Geometry: final body of the model. Coordinates: model frame, mm. Face numbers are marked on the shaded views. A direction names the side the tool comes from. Give positions to 0.01 mm unless a question says otherwise; leave off trailing zeros. Order: outer loops, then holes, each group sorted by start corner. A loop starts at its lowest first (then second) coordinate and runs counter-clockwise, first axis right, second up. Notation, with made-up numbers: (18.5, 64.25) - (26.5, 64.25) arc R31 cw to (26.5, 99.25) - close; hole circle Ø8 at (18.5, 85). An arc over 180 degrees is marked (long way). One line per item, written item: value.
```python
from build123d import *

# Parameters (mm, degrees)
SKETCH_1_R          = 1.149999389
SKETCH_1_R_2        = 1.149999553
SKETCH_1_R_3        = 1.149999359
SKETCH_1_R_4        = 1.149997552
EXTRUDE_1_DEPTH     = 3
SKETCH_4_W          = 12.999996185
SKETCH_4_H          = 4.628
SKETCH_4_W_2        = 13.000000328
EXTRUDE_2_DEPTH     = 12.361
SKETCH_6_R          = 1
CUT_EXTRUDE_2_DEPTH = 200


with BuildPart() as part:
    # 草图1 → 凸台-拉伸1 (new body)
    with BuildSketch(Plane.XY):
        Polygon((13.161137581, 10.828393936), (13.161137581, -17.026895523), (51.838863373, -17.026895523), (51.838863373, 10.828393936), (64.838859558, 10.828393936), (64.838859558, -16.700000763), (73.376037598, -16.700000763), (73.376037598, -23.38126564), (-8.376040459, -23.38126564), (-8.376040459, -16.700000763), (0.161137253, -16.700000763), (0.161137253, 10.828393936), align=None)
        with Locations((-2.800555034, -20.040632255)):
            Circle(SKETCH_1_R, mode=Mode.SUBTRACT)
        with Locations((8.199444431, -20.040632183)):
            Circle(SKETCH_1_R_2, mode=Mode.SUBTRACT)
        with Locations((56.800554471, -20.040632944)):
            Circle(SKETCH_1_R_3, mode=Mode.SUBTRACT)
        with Locations((67.800554915, -20.040625058)):
            Circle(SKETCH_1_R_4, mode=Mode.SUBTRACT)
    extrude(amount=EXTRUDE_1_DEPTH)

    # 草图4 → 凸台-拉伸2 (add)
    with BuildSketch(Plane(origin=(0, 0, 0), x_dir=(-1, 0, 0), z_dir=(0, 0, -1))):
        with Locations((-58.338861466, 8.514393936)):
            Rectangle(SKETCH_4_W, SKETCH_4_H)
        with Locations((-6.661137417, 8.514393936)):
            Rectangle(SKETCH_4_W_2, SKETCH_4_H)
    extrude(amount=EXTRUDE_2_DEPTH)

    # 草图6 → 切除-拉伸2 (cut)
    with BuildSketch(Plane(origin=(64.838859558, 0, 0), x_dir=(0, 0, -1), z_dir=(1, 0, 0))):
        with Locations((6.361, 8.828393936)):
            Circle(SKETCH_6_R)
    extrude(amount=-CUT_EXTRUDE_2_DEPTH, mode=Mode.SUBTRACT)


solid = part.part
```
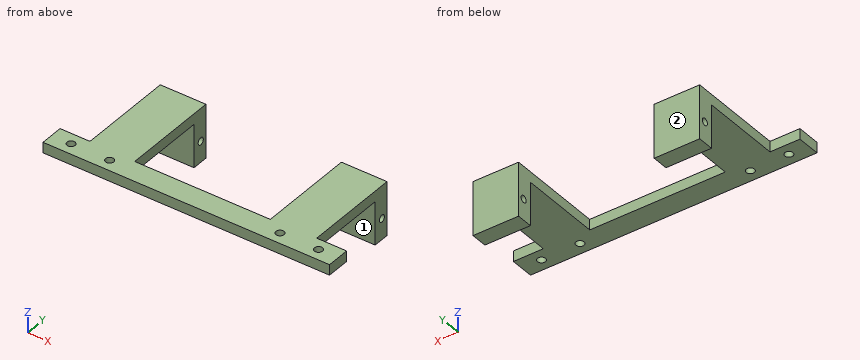
1) Section C-C, the plane x = 63. Return loops of the section in (y, z).
Answers below:
outline: (-23.38, 0) - (6.2, 0) - (6.2, -12.36) - (10.83, -12.36) - (10.83, 3) - (-23.38, 3) - close; hole circle Ø2 at (8.83, -6.36)
2) Material intervals for line 1 along X through (y, z) = (7, -5.5); line 2 along Y through (x, z) = (12, -5); line 3 along Z through (x, y) = (11.5, -4), sorted ascending.
Answers below:
line 1: 0.16 to 13.16, 51.84 to 64.84
line 2: 6.2 to 10.83
line 3: 0 to 3
3) Section B-B, the plane z = -11. Return loops of the section in (x, y), then the cut area to 3 significant figures.
Answers below:
outline: (0.16, 6.2) - (13.16, 6.2) - (13.16, 10.83) - (0.16, 10.83) - close; (51.84, 6.2) - (64.84, 6.2) - (64.84, 10.83) - (51.84, 10.83) - close
area: 120 mm^2
4) Section D-D, the plane z = 1.75. Return loops of the section in (x, y), then the cut area to 3 significant figures.
Answers below:
outline: (-8.38, -23.38) - (73.38, -23.38) - (73.38, -16.7) - (64.84, -16.7) - (64.84, 10.83) - (51.84, 10.83) - (51.84, -17.03) - (13.16, -17.03) - (13.16, 10.83) - (0.16, 10.83) - (0.16, -16.7) - (-8.38, -16.7) - close; hole circle Ø2.3 at (-2.8, -20.04); hole circle Ø2.3 at (8.2, -20.04); hole circle Ø2.3 at (56.8, -20.04); hole circle Ø2.3 at (67.8, -20.04)
area: 1,230 mm^2
5) First-contact query: pin 1 (3 mm diameter, centred on x = 8.2, y = -20.04, fed in from -Z); pin 2 (2 mm diameter, centred on x = 56.8, y = -20.04, fed in from +Z); pin 3 (1.5 mm diameter, centred on y = -11.5, z = 0.5, fed in from -X); pin 4 (6 mm diameter, centred on x = 57, z = -3.5, fed in from -Y). Flat tips, straight axial feed; report the tip coordinate or a pass-through.
Answers below:
pin 1: z = 0
pin 2: through
pin 3: x = 0.16
pin 4: y = 6.2
6) Section A-A, the plane y = 1.5. Return loops of the section in (x, z), then the cut area to 3 significant figures.
Answers below:
outline: (0.16, 0) - (13.16, 0) - (13.16, 3) - (0.16, 3) - close; (51.84, 0) - (64.84, 0) - (64.84, 3) - (51.84, 3) - close
area: 78.0 mm^2
7) Set-up query: the marked faces 1 and 2. Return all of +Z, -Z, +X, -X, +Y, -Y with unobstructed straight access to the full face (end or side cutting, diameter ignored); none if empty.
Answers below:
face 1: -Z, +X, -X, -Y
face 2: +Z, -Z, +X, -X, +Y
